```python
from build123d import *

# Parameters (mm, degrees)
SKETCH1_W           = 180
SKETCH1_H           = 180
BOSS_EXTRUDE1_DEPTH = 3
FILLET1_R           = 10
SKETCH2_R           = 1.7
CUT_EXTRUDE1_DEPTH  = 3
SKETCH3_R           = 4
CUT_EXTRUDE2_DEPTH  = 128.314571044


with BuildPart() as part:
    # Sketch1 → Boss-Extrude1 (new body)
    with BuildSketch(Plane(origin=(0, 0, 0), x_dir=(1, 0, 0), z_dir=(0, 1, 0))):
        Rectangle(SKETCH1_W, SKETCH1_H)
    extrude(amount=BOSS_EXTRUDE1_DEPTH)

    # Fillet1
    fillet1_edges = [part.edges().sort_by_distance(p)[0] for p in [
        (90, 1.5, 90),
        (-90, 1.5, 90),
        (-90, 1.5, -90),
        (90, 1.5, -90),
    ]]
    fillet(fillet1_edges, radius=FILLET1_R)

    # Sketch2 → Cut-Extrude1 (cut)
    with BuildSketch(Plane(origin=(0, 3, 0), x_dir=(1, 0, 0), z_dir=(0, 1, 0))):
        with Locations(Location((-82, 75, 0), (0, 0, 270))):
            Circle(SKETCH2_R)
        with Locations(Location((-68, 75, 0), (0, 0, 270))):
            Circle(SKETCH2_R)
        with Locations(Location((68, 75, 0), (0, 0, 270))):
            Circle(SKETCH2_R)
        with Locations(Location((82, 75, 0), (0, 0, 270))):
            Circle(SKETCH2_R)
        with Locations(Location((-82, -75, 0), (0, 0, 270))):
            Circle(SKETCH2_R)
        with Locations(Location((-68, -75, 0), (0, 0, 270))):
            Circle(SKETCH2_R)
        with Locations(Location((68, -75, 0), (0, 0, 270))):
            Circle(SKETCH2_R)
        with Locations(Location((82, -75, 0), (0, 0, 270))):
            Circle(SKETCH2_R)
        with Locations(Location((-54, -75, 0), (0, 0, 270))):
            Circle(SKETCH2_R)
        with Locations(Location((54, -75, 0), (0, 0, 270))):
            Circle(SKETCH2_R)
        with Locations(Location((-40, -75, 0), (0, 0, 270))):
            Circle(SKETCH2_R)
        with Locations(Location((40, -75, 0), (0, 0, 270))):
            Circle(SKETCH2_R)
    extrude(amount=-CUT_EXTRUDE1_DEPTH, mode=Mode.SUBTRACT)

    # Sketch3 → Cut-Extrude2 (cut, through all)
    with BuildSketch(Plane(origin=(0, 3, 0), x_dir=(1, 0, 0), z_dir=(0, 1, 0))):
        with Locations(Location((40, 45, 0), (0, 0, 270))):
            Circle(SKETCH3_R)
    extrude(amount=-CUT_EXTRUDE2_DEPTH, mode=Mode.SUBTRACT)


solid = part.part
```
Geometry check sheet. Reference: the model listing, model coordinates, mm. Coordinates: 2 decimals unless noted, no trailing zeros. Order: outer loops, then holes, each group sorted by start corner. A loop starts at its lowest first (then second) coordinate and runs counter-clockwise, first axis right, second up.
Item 1: Depth check by flat-ended pin: pin 1 (2.5 mm diameter, centred on x = -68, z = 75, fed in from -Y); pin 2 (4.5 mm diameter, centred on x = -82, z = 75, fed in from +Y). Enter the tip coordinate at first touch or a pass-through.
Item 2: Section check A-A (z = -46.5). Enter the section's corners in (x, y).
Item 3: Mould release check, pull along Z, two halves, no side actions. Record for faces 1 (the cylindrical face through (43.966, 1.521, -45.521)), 2 (the cylindrical face through (-87.15, 1.52, 86.99)), 3 (the flat face through (-1, 3, -1)), 4 (the cylindrical face through (87.15, 1.52, -86.99)): released by +Z, released by -Z, zero draft, split by the parting line, or undercut.
Item 4: Scan lines: line 1 along Z through (x, y) = (68, 0.6); line 2 along X through (y, z) = (1.5, -75); line 3 along X through (y, z) = (1.6, -45). Record each from-to range of solid material in increasing order.
Check sheet entries:
1. pin 1: passes through
1. pin 2: stops at y = 3
2. outline: (-90, 0) - (36.29, 0) - (36.29, 3) - (-90, 3) - close; (43.71, 0) - (90, 0) - (90, 3) - (43.71, 3) - close
3. face 1: undercut
3. face 2: released by +Z
3. face 3: zero draft
3. face 4: released by -Z
4. line 1: z = -90 to -76.7, -73.3 to 73.3, 76.7 to 90
4. line 2: x = -90 to -83.7, -80.3 to -69.7, -66.3 to 66.3, 69.7 to 80.3, 83.7 to 90
4. line 3: x = -90 to 36, 44 to 90
